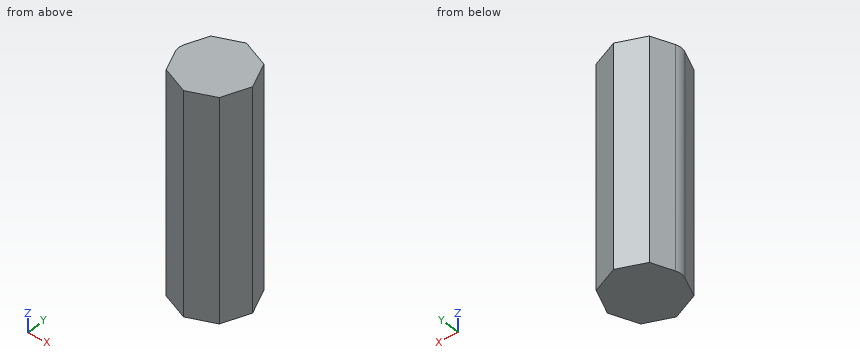
from build123d import *

# Parameters (mm, degrees)
F1_DEPTH = 300
F2_R     = 20


with BuildPart() as f1:
    # F0 (on Top) → F1 (new body)
    with BuildSketch(Plane.XY):
        Polygon((35.661297, 35.661297), (0, 50.432689), (-35.661297, 35.661297), (-50.432689, 0), (-35.661297, -35.661297), (0, -50.432689), (35.661297, -35.661297), (50.432689, 0), align=None)
    extrude(amount=F1_DEPTH)

    # F2
    f2_edges = [f1.edges().sort_by_distance(p)[0] for p in [
        (-50.432689, 0, 150),
    ]]
    fillet(f2_edges, radius=F2_R)


solid = f1.part
The listing builds one solid part. Answer for the finished solid, in the listing's coordinates (mm). Give positions to 0.01 mm unless a question says otherwise; leave off trailing zeros. Write each loop counter-clockwise with the first axis right and the second up, starting at its lowest first coordinate (ties: lowest second). Pieces come first, ordered by that corner, then holes. Notation, with made-up numbers: (42.25, 19) - (83.25, 19) arc R23 cw to (83.25, 46) - close; hole circle Ø5 at (58.25, 34.25). An arc over 180 degrees is marked (long way). Use a Markdown table: item, result.
1. Section A-A on z = 209.5 is taken. Write down the section's boundary in (x, y), plus the area to 3 significant figures.
Values follow:
| item | result |
|---|---|
| outline | (-47.26, -7.65) - (-35.66, -35.66) - (0, -50.43) - (35.66, -35.66) - (50.43, 0) - (35.66, 35.66) - (0, 50.43) - (-35.66, 35.66) - (-47.26, 7.65) arc R20 ccw to start |
| area | 7,190 mm² |
2. Section B-B on y = -13 is taken. Write down the section's boundary in (x, z), plus the area to 3 significant figures.
Values follow:
| item | result |
|---|---|
| outline | (-45.05, 0) - (45.05, 0) - (45.05, 300) - (-45.05, 300) - close |
| area | 27,000 mm² |
3. Each of these flat-tipped pins is pushed along its axis until it touches: P1, Ø2, axis at y = 16, z = 154, coming from the -X side; P2, Ø12, axis at y = 34, z = 211.5, coming from the -X side; P3, Ø8, axis at x = -16.5, z = 56.5, coming from the +Y side (3 decimals); P4, Ø6, axis at x = 15, y = 26.5, coming from the -Z side. Where does it stop, or does it pass through?
Values follow:
| item | result |
|---|---|
| P1 | stops at x = -44.22 |
| P2 | stops at x = -38.83 |
| P3 | stops at y = 45.255 |
| P4 | stops at z = 0 |
4. Section C-C on x = -29 is taken. Write down the section's boundary in (y, z).
Values follow:
| item | result |
|---|---|
| outline | (-38.42, 0) - (38.42, 0) - (38.42, 300) - (-38.42, 300) - close |
5. Find the intervals of material crossed by probe 1 along Y at (x, z) = (-14, 207); probe 2 along Y at (x, z) = (-7, 232); probe 3 along X at (y, z) = (41, 230.5), in increasing order. Write a range as from..to.
Values follow:
| item | result |
|---|---|
| probe 1 | y = -44.63..44.63 |
| probe 2 | y = -47.53..47.53 |
| probe 3 | x = -22.77..22.77 |
